```python
from build123d import *

# Parameters (mm, degrees)
F0_R        = 1.27
F1_DEPTH    = 88.9
F5_T1_DEPTH = 181.4661742094


# Not quite as in the source:
# - a fillet or chamfer that OpenCascade refuses, or shapes differently, is made with other operations: its cross-section is extruded or revolved along the edge and cut away or added


with BuildPart() as f1:
    # F0 (on Front) → F1 (new body, symmetric)
    with BuildSketch(Plane.XZ):
        Polygon((4.0324625191, -0.0515205351), (2.0608493518, 3.4664547138), (-1.9716131673, 3.5179752489), (-4.0324625191, 0.0515205351), (-2.0608493518, -3.4664547138), (1.9716131673, -3.5179752489), align=None)
        Circle(F0_R, mode=Mode.SUBTRACT)
    extrude(amount=F1_DEPTH, both=True)

    # F2 (on Top) → F4 (revolve, cut)
    with BuildSketch(Plane.XY):
        Polygon((0, -99.6820554137), (0, -88.9), (-4.0324625191, -74.2031688439), (-4.0324625191, -99.6820554137), align=None)
    revolve(axis=Axis((0, -76.0434828699, 0), (0, -1, 0)), mode=Mode.SUBTRACT)

    # F5: fillet of radius 1.27 on 6 edges, made by hand

    # F5_s2 → F5_t1 (cut)
    with BuildSketch(Plane.XZ.offset(-90.7330871047)):
        with BuildLine():
            ThreePointArc((2.4193244731, 2.8268228503), (1.960448821, 3.2975758517), (1.3276743483, 3.4758220838))
            Line((1.3276743483, 3.4758220838), (2.0608493518, 3.4664547138))
            Line((2.0608493518, 3.4664547138), (2.4193244731, 2.8268228503))
        make_face()
        with BuildLine():
            ThreePointArc((-1.2384381638, 3.5086078789), (-1.875560048, 3.3465864076), (-2.3463130494, 2.8877107555))
            Line((-2.3463130494, 2.8877107555), (-1.9716131673, 3.5179752489))
            Line((-1.9716131673, 3.5179752489), (-1.2384381638, 3.5086078789))
        make_face()
        with BuildLine():
            ThreePointArc((-3.6739873978, -0.5881113283), (-3.836008869, 0.0490105559), (-3.6577626369, 0.6817850286))
            Line((-3.6577626369, 0.6817850286), (-4.0324625191, 0.0515205351))
            Line((-4.0324625191, 0.0515205351), (-3.6739873978, -0.5881113283))
        make_face()
        with BuildLine():
            ThreePointArc((-1.3276743483, -3.4758220838), (-1.960448821, -3.2975758517), (-2.4193244731, -2.8268228503))
            Line((-2.4193244731, -2.8268228503), (-2.0608493518, -3.4664547138))
            Line((-2.0608493518, -3.4664547138), (-1.3276743483, -3.4758220838))
        make_face()
        with BuildLine():
            ThreePointArc((2.3463130494, -2.8877107555), (1.875560048, -3.3465864076), (1.2384381638, -3.5086078789))
            Line((1.2384381638, -3.5086078789), (1.9716131673, -3.5179752489))
            Line((1.9716131673, -3.5179752489), (2.3463130494, -2.8877107555))
        make_face()
        with BuildLine():
            ThreePointArc((3.6577626369, -0.6817850286), (3.836008869, -0.0490105559), (3.6739873978, 0.5881113283))
            Line((3.6739873978, 0.5881113283), (4.0324625191, -0.0515205351))
            Line((4.0324625191, -0.0515205351), (3.6577626369, -0.6817850286))
        make_face()
    extrude(amount=F5_T1_DEPTH, mode=Mode.SUBTRACT)


solid = f1.part
```
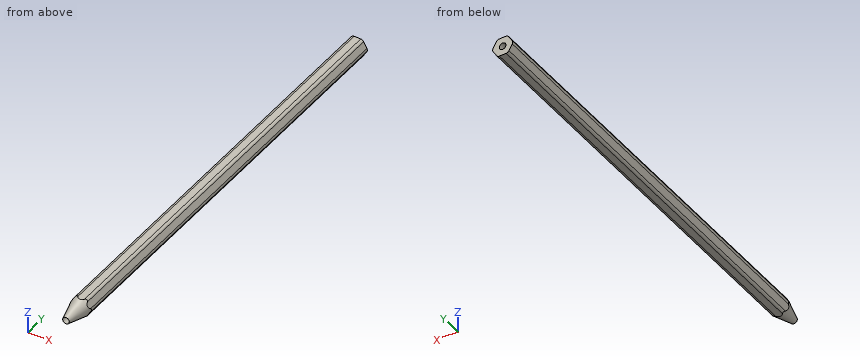
Part model, mm, in its own coordinate system. Give positions to 0.01 mm unless a question says otherwise; leave off trailing zeros. Write each loop counter-clockwise with the first axis right and the second up, starting at its lowest first coordinate (ties: lowest second). Pieces come first, ordered by that corner, then holes. Notation, with made-up numbers: M 16,79 L 47,79 A11 cw 47,84 Z; hole C -10.75,-18.75 d2. An arc over 180 degrees is marked long. Use CSV: the item, a comma, the result in double quotes.
Item 1: Drill centre lines: probe 1 along Z at (x, y) = (0, 27); probe 2 along X at (y, z) = (18.5, 0); probe 3 along Z at (x, y) = (-0.25, 66.5). Where is each one in solid material? Low to high.
Taken from the geometry:
probe 1,"z = -3.49 to -1.27, 1.27 to 3.49"
probe 2,"x = -3.84 to -1.27, 1.27 to 3.84"
probe 3,"z = -3.49 to -1.25, 1.25 to 3.5"
Item 2: Slice it at A-A on y = 13.5. Write the cut outline in (x, z), plus the area to 3 significant figures.
Taken from the geometry:
outline,"M -3.67,-0.59 L -2.42,-2.83 A1.27 ccw -1.33,-3.48 L 1.24,-3.51 A1.27 ccw 2.35,-2.89 L 3.66,-0.68 A1.27 ccw 3.67,0.59 L 2.42,2.83 A1.27 ccw 1.33,3.48 L -1.24,3.51 A1.27 ccw -2.35,2.89 L -3.66,0.68 A1.27 ccw Z; hole C 0,0 d2.54"
area,"36.7 mm²"
Item 3: Slice it at B-B on x = 0. Write the cut outline in (y, z), plus the area to 3 significant figures.
Taken from the geometry:
outline,"M -84.27,-1.27 L -76.17,-3.49 L 88.9,-3.49 L 88.9,-1.27 Z; M -84.27,1.27 L 88.9,1.27 L 88.9,3.49 L -76.17,3.49 Z"
area,"752 mm²"
